from build123d import *

# Parameters (mm, degrees)
CYLINDER029_R           = 2
CYLINDER029_DEPTH       = 8
CYLINDER029_PITCH_ANGLE = 90
ARRAY027_Z_COUNT        = 2
ARRAY027_Z_PITCH        = 30
BOX017_W                = 8
BOX017_H                = 40
BOX017_DEPTH            = 50


with BuildPart() as array027:
    # Cylinder029 → Cylinder029 (new body)
    with BuildSketch(Plane.XY):
        Circle(CYLINDER029_R)
    extrude(amount=CYLINDER029_DEPTH)


with BuildPart() as array027_1:
    # Cylinder029 pitch: moved
    add(array027.part.rotate(Axis((0, 0, 0), (0, 1, 0)), CYLINDER029_PITCH_ANGLE))


with BuildPart() as array027_2:
    # Cylinder029 placement: moved
    add(array027_1.part.moved(Location((144, -87, -14))))

    # Array027 Z: Array027 ×2


with BuildPart() as array027_3:
    add(array027_2.part)
    with Locations(*[(0, 0, -i * ARRAY027_Z_PITCH) for i in range(1, ARRAY027_Z_COUNT)]):
        add(array027_2.part)


with BuildPart() as case_2_con005:
    # Box017 → Box017 (new body)
    with BuildSketch(Plane(origin=(144, -107, -54), x_dir=(1, 0, 0), z_dir=(0, 0, 1))):
        with Locations((4, 20)):
            Rectangle(BOX017_W, BOX017_H)
    extrude(amount=BOX017_DEPTH)

    # Cut028: cut Array027
    add(array027_3.part, mode=Mode.SUBTRACT)


solid = case_2_con005.part
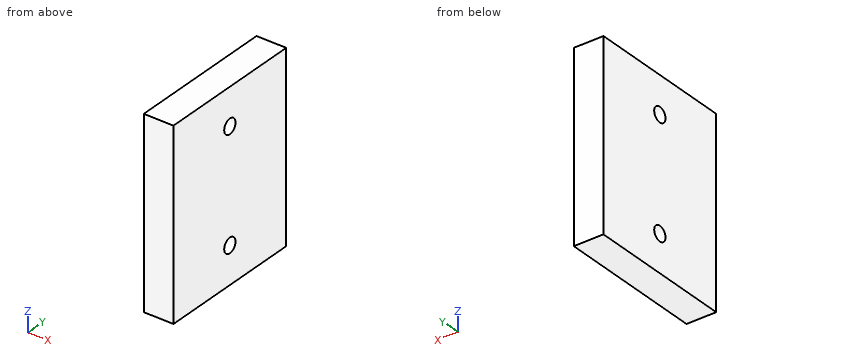
Check sheet for the modelled part. Datum: model origin and axes. Units: mm. Coordinates: 2 decimals unless noted, no trailing zeros. Loops run counter-clockwise (first coordinate to the right, second up) from the corner with the lowest first, then second, coordinate; pieces in that order, holes last. Notation, with made-up numbers: (-37.75, 68) -> (17.25, 68) arc R29 ccw to (17.25, 99) -> close; hole circle Ø1 at (77.25, 50.25). An arc over 180 degrees is marked (long way). Answer in a Markdown table with one row per item.
1. Material ranges on line 1 along Y through (x, z) = (150.75, -14); line 2 along Z through (x, y) = (150, -88), recorded low to high. Write a range as [from, to].
Check values:
| item | result |
|---|---|
| line 1 | y = [-107, -89], [-85, -67] |
| line 2 | z = [-54, -45.73], [-42.27, -15.73], [-12.27, -4] |
2. Sectioned sample at A-A, the plane y = -87. Record the boundary of the cut face in (x, z), then the cut area to 3 significant figures.
Check values:
| item | result |
|---|---|
| outline | (144, -54) -> (152, -54) -> (152, -46) -> (144, -46) -> close; (144, -42) -> (152, -42) -> (152, -16) -> (144, -16) -> close; (144, -12) -> (152, -12) -> (152, -4) -> (144, -4) -> close |
| area | 336 mm2 |
3. Sectioned sample at B-B, the plane z = -44. Record the boundary of the cut face in (x, y), then the cut area to 3 significant figures.
Check values:
| item | result |
|---|---|
| outline | (144, -107) -> (152, -107) -> (152, -89) -> (144, -89) -> close; (144, -85) -> (152, -85) -> (152, -67) -> (144, -67) -> close |
| area | 288 mm2 |
